Can you work these out from the model? Positions are in its coordinate system, mm. A direction names the side the tool comes from. Coordinates: 2 decimals unless noted, no trailing zeros. Order: outer loops, then holes, each group sorted by start corner. A loop starts at its lowest first (then second) coordinate and runs counter-clockwise, first axis right, second up. Notation, with made-up numbers: (17.5, 51) -> (26.5, 51) arc R17 ccw to (26.5, 66) -> close; hole circle Ø4 at (51.25, 34). An arc over 180 degrees is marked (long way). Return JSON: item names as keys, results as strings. Group by question number.
1) For faces 1 (the flat face through (32.5, 96, -10)), 2 (the flat face through (196, 5.5, 82)), 3 (the flat face through (13, 86.5, -8)), 4 (the flat face through (67, 97, -20)), 5 (the flat face through (174, 96, -15)), which set-ups out of +Z, -Z, +X, -X, +Y, -Y let a thin tool reach every point of the face, with its end or its side?
2) If we section it at B-B, the plane x = 66: Please give me the cut outline in (y, z).
3) If we section it at C-C, the plane y = -65.5: Please give me the cut outline in (x, z), then the cut area to 3 significant figures.
4) Thinking about a two-plate mould opening in X: for faces 6 (the flat face through (215, -2, -167)), 7 (the flat face through (-196.724, -59.753, 21.195)), 8 (the flat face through (177.5, -17, 36)), which applies, +X half, -X half, draft (parallel to the pull), parting line (faces both ways), or undercut?
5) If we section it at A-A, the plane z = 58.5: Please give me the cut outline in (x, y).
6) If we section it at D-D, the plane z = -92.5: Please give me the cut outline in (x, y).
7) If I drill on probe 1 along X at (y, z) = (-13, 76); probe 2 along X at (y, z) = (-4.5, 11.5); probe 3 along Y at (x, z) = (208, -19), over which ranges is the centre line in solid material (lowest first)? Write a range as from..to.
8) For pin 1 (5 mm diameter, centred on x = 206.5, y = -84.5, fed in from -Z); pin 2 (5 mm diameter, centred on x = 47.5, y = 18, fed in from +Z); pin 3 (10 mm diameter, centred on y = 103, z = -5.5, fed in from -X); pin 4 (1.5 mm diameter, centred on x = -11, z = 1.5, fed in from -Y), each with a flat end and sliding along its axis, tell me the tip position at first contact or that it passes through.
Autodesk Inventor part; units mm, degrees
ref_plane "YZ Plane" through (0, 0, 0) normal (1, 0, 0) x (0, 1, 0)
ref_plane "XZ Plane" through (0, 0, 0) normal (0, 1, 0) x (-1, 0, 0)
ref_plane "XY Plane" through (0, 0, 0) normal (0, 0, 1) x (1, 0, 0)
sketch "Sketch1" plane through (0, 0, 0) normal (0, 0, 1) x (1, 0, 0)
  line L0 (-212.5, -81.5) -> (212.5, -81.5)
  line L1 (212.5, -81.5) -> (212.5, 81.5)
  line L2 (212.5, 81.5) -> (-212.5, 81.5)
  line L3 (-212.5, 81.5) -> (-212.5, -81.5)
  line L4 (-212.5, -81.5) -> (212.5, 81.5) construction
  line L5 (212.5, -81.5) -> (-212.5, 81.5) construction
  point P0 (0, 0)
  dimension "d0" = 163
  dimension "d1" = 425
extrude "Extrusion1" add sketch "Sketch1" against normal blind 335
sketch "Sketch2" plane through (-212.5, -81.5, 0) normal (0, -1, 0) x (1, 0, 0)
  line L0 (0, 0) -> (425, 0) construction
  line L1 (425, -8) -> (409.5, -8)
  line L2 (409.5, -8) -> (409.5, -28)
  line L3 (409.5, -28) -> (425, -28)
  line L4 (425, -28) -> (425, -8)
  line L5 (20, -10) -> (0, -10)
  line L6 (0, -10) -> (0, -25.5)
  line L7 (0, -25.5) -> (20, -25.5)
  line L8 (20, -25.5) -> (20, -10)
  line L9 (0, -10) -> (0, 0) construction
  line L10 (425, -8) -> (425, 0) construction
  point P0 (212.5, 0)
  dimension "d4" = 8
  dimension "d5" = 10
  dimension "d6" = 15.5
  dimension "d7" = 20
  dimension "d8" = 15.5
  dimension "d9" = 20
extrude "Extrusion2" add sketch "Sketch2" along normal blind 6
sketch "Sketch3" plane through (212.5, -81.5, 0) normal (1, 0, 0) x (0, 0, -1)
  line L0 (0, 0) -> (0, 163)
  line L1 (0, 0) -> (-5, 0)
  line L2 (-5, 0) -> (-40, 47)
  line L3 (-40, 47) -> (-90, 47)
  line L4 (-90, 47) -> (-90, 87)
  line L5 (-90, 87) -> (-69, 87)
  line L6 (-69, 93) -> (-34.909, 105.3518)
  line L7 (-69, 87) -> (-69, 93)
  arc A0 (-34.909, 105.3518) -> (-5, 148) centre (-50.3612, 148) ccw
  line L8 (-34.909, 105.3518) -> (0, 118) construction
  arc A1 (-37.8496, 44.1124) -> (-43.6003, 47) centre (-43.6003, 39.8299) ccw
  line L9 (-5, 148) -> (-5, 163)
  line L10 (-5, 163) -> (0, 163)
  dimension "d12" = 5
  dimension "d13" = 47
  dimension "d14" = 35
  dimension "d15" = 40
  dimension "d16" = 90
  dimension "d17" = 118
  dimension "d18" = 93
  dimension "d19" = 69
  dimension "d23" = 55
  dimension "d26" = 5
  dimension "d27" = 15
extrude "Extrusion3" add sketch "Sketch3" against normal blind 35
sketch "Sketch4" plane through (-212.5, -81.5, 0) normal (-1, 0, 0) x (0, 0, 1)
  line L0 (0, 0) -> (0, 163)
  line L1 (0, 0) -> (5, 0)
  line L2 (5, 0) -> (37.8496, 44.1124)
  arc A0 (43.6003, 47) -> (37.8496, 44.1124) centre (43.6003, 39.8299) ccw
  line L3 (43.6003, 47) -> (90, 47)
  line L4 (90, 47) -> (90, 87)
  line L5 (90, 87) -> (69, 87)
  line L6 (69, 87) -> (69, 93)
  line L7 (69, 93) -> (34.909, 105.3518)
  arc A1 (5, 148) -> (34.909, 105.3518) centre (50.3612, 148) ccw
  line L8 (5, 148) -> (5, 163)
  line L9 (5, 163) -> (0, 163)
  point P0 (0, 81.5)
extrude "Extrusion4" add sketch "Sketch4" against normal blind 32
sketch "Sketch5" plane through (-212.5, 81.5, -335) normal (0, 1, 0) x (1, 0, 0)
  line L0 (390, -335) -> (32, -335)
  line L1 (32, -335) -> (8, -335)
  line L2 (8, -335) -> (8, -330)
  line L3 (8, -330) -> (39, -330)
  line L4 (39, -330) -> (39, -335)
  line L5 (0, 0) -> (0, -340) construction
  point P0 (212.5, -335)
  dimension "d28" = 39
  dimension "d29" = 5
  dimension "d30" = 8
extrude "Extrusion5" add sketch "Sketch5" along normal blind 30
sketch "Sketch6" plane through (-212.5, 81.5, -335) normal (0, 1, 0) x (1, 0, 0)
  line L0 (0, 0) -> (0, -340) construction
  line L1 (390, -335) -> (39, -335)
  line L2 (212, -335) -> (212, -315)
  line L3 (212, -315) -> (240, -315)
  line L4 (240, -315) -> (240, -335)
  point P0 (212.5, -335)
  dimension "d33" = 212
  dimension "d34" = 240
  dimension "d35" = 20
extrude "Extrusion6" add sketch "Sketch6" along normal blind 5
sketch "Sketch7" plane through (0, 0, 0) normal (0, 0, 1) x (1, 0, 0)
  line L0 (177.5, 81.5) -> (27.5, 81.5)
  line L1 (32.5, 81.5) -> (32.5, 111.5)
  line L2 (-212.5, -81.5) -> (-212.5, 81.5) construction
  line L3 (102.5, 81.5) -> (102.5, 111.5)
  line L4 (32.5, 111.5) -> (102.5, 111.5)
  point P0 (0, 0)
  dimension "d38" = 245
  dimension "d39" = 315
  dimension "d40" = 30
extrude "Extrusion7" add sketch "Sketch7" against normal blind 20
sketch "Sketch8" plane through (-212.5, 81.5, -335) normal (0, 1, 0) x (1, 0, 0)
  line L0 (0, 0) -> (0, -340) construction
  line L1 (374, -315) -> (399, -315)
  line L2 (399, -315) -> (399, -320)
  line L3 (399, -320) -> (374, -320)
  line L4 (374, -320) -> (374, -315)
  line L5 (390, -335) -> (315, -335) construction
  point P0 (212.5, -335)
  dimension "d43" = 374
  dimension "d44" = 399
  dimension "d45" = 15
  dimension "d46" = 20
extrude "Extrusion8" add sketch "Sketch8" along normal blind 30
sketch "Sketch9" plane through (-212.5, 86.5, -335) normal (0, 1, 0) x (1, 0, 0)
  line L0 (240, -315) -> (212, -315)
  line L1 (240, -335) -> (240, -315)
  line L2 (212, -320) -> (240, -320)
  line L3 (212, -315) -> (212, -320)
  line L4 (8, -330) -> (8, -335) construction
  point P0 (212.5, -335)
extrude "Extrusion9" add sketch "Sketch9" along normal up to surface (25 mm away)
sketch "Sketch10" plane through (-212.5, 5.5, 90) normal (0, 1, 0) x (1, 0, 0)
  line L0 (0, 0) -> (32, 0)
  line L1 (425, 0) -> (390, 0)
  circle A0 centre (16, 14) radius 4
  circle A1 centre (407.5, 14) radius 4
  line L2 (390, 0) -> (407.5, 14) construction
  line L3 (407.5, 14) -> (425, 0) construction
  line L4 (32, 0) -> (16, 14) construction
  line L5 (16, 14) -> (0, 0) construction
  line L6 (16, 14) -> (407.5, 14) construction
  point P0 (212.5, 90)
  dimension "d51" = 8
  dimension "d52" = 14
extrude "Extrusion10" cut sketch "Sketch10" against normal up to surface (40 mm away)
sketch "Sketch11" plane through (212.5, -81.5, -335) normal (1, 0, 0) x (0, 0, -1)
  line L0 (-327, -6) -> (-327, 0)
  line L1 (-327, 0) -> (-340, 0)
  line L2 (-340, 0) -> (-372.8496, 44.1124)
  arc A0 (-372.8496, 44.1124) -> (-378.6003, 47) centre (-378.6003, 39.8299) ccw
  line L3 (-378.6003, 47) -> (-425, 47)
  line L4 (-425, 47) -> (-425, 87)
  line L5 (-425, 87) -> (-404, 87)
  line L6 (-404, 87) -> (-404, 93)
  line L7 (-404, 93) -> (-369.909, 105.3518)
  arc A1 (-369.909, 105.3518) -> (-340, 148) centre (-385.3612, 148) ccw
  line L8 (-340, 148) -> (-340, 163)
  line L9 (-340, 163) -> (0, 163)
  line L10 (0, 163) -> (0, 0)
  line L11 (0, 0) -> (-307, 0)
  line L12 (-307, 0) -> (-307, -6)
  line L13 (-307, -6) -> (-327, -6)
  point P0 (-335, 81.5)
extrude "Extrusion11" add sketch "Sketch11" along normal blind 2.5
sketch "Sketch12" plane through (215, -81.5, -335) normal (1, 0, 0) x (0, 0, -1)
  line L0 (-415, 87) -> (-407, 87) construction
  line L1 (-411, 87) -> (-411, 3) construction
  line L2 (-411, 3) -> (-316, 3) construction
  line L3 (-316, 3) -> (-169, 3) construction
  line L4 (-169, 3) -> (-22, 3) construction
  circle A0 centre (-316, 3) radius 3
  circle A1 centre (-169, 3) radius 3
  circle A2 centre (-22, 3) radius 3
  line L5 (-327, -6) -> (-307, -6)
  point P0 (-335, 81.5)
  dimension "d57" = 95
  dimension "d58" = 242
  dimension "d59" = 389
  dimension "d60" = 6
  dimension "d63" = 9
extrude "Extrusion12" cut sketch "Sketch12" against normal blind 10
properties part number "IMA Battery Case Primitive"
Result sheet:
{
 "1": {"face 1": "+Z, -Z, +Y", "face 2": "+Z, +X, -X, +Y", "face 3": "+Z, +Y", "face 4": "-Z, +X, -X, +Y", "face 5": "+Z, +X, +Y"},
 "2": {"outline": "(-81.5, -335) -> (81.5, -335) -> (81.5, -20) -> (111.5, -20) -> (111.5, 0) -> (-81.5, 0) -> close"},
 "3": {"outline": "(-212.5, -335) -> (215, -335) -> (215, 16.91) -> (177.5, 16.91) -> (177.5, 0) -> (-180.5, 0) -> (-180.5, 16.91) -> (-212.5, 16.91) -> close", "area": "144,000 mm2"},
 "4": {"face 6": "+X half", "face 7": "draft", "face 8": "undercut"},
 "5": {"outline": "(-212.5, -34.5) -> (-180.5, -34.5) -> (-180.5, 15.3) -> (-212.5, 15.3) -> close; (177.5, -34.5) -> (215, -34.5) -> (215, 15.3) -> (177.5, 15.3) -> close"},
 "6": {"outline": "(-212.5, -81.5) -> (215, -81.5) -> (215, 81.5) -> (-212.5, 81.5) -> close"},
 "7": {"probe 1": "x = -212.5..-200.5, -192.5..-180.5, 177.5..191, 199..215", "probe 2": "x = -212.5..-180.5, 177.5..215", "probe 3": "y = -87.5..-81.5, -75.5..81.5"},
 "8": {"pin 1": "stops at z = -28", "pin 2": "stops at z = 0", "pin 3": "stops at x = -204.5", "pin 4": "passes through"}
}
